Design review of the part built by this model. Coordinates are the model's own, in mm. Face numbers are marked on the shaded views. Round coordinates to 2 decimals unless told otherwise and drop trailing zeros. Order: outer loops, then holes, each group sorted by start corner. A loop starts at its lowest first (then second) coordinate and runs counter-clockwise, first axis right, second up. Notation, with made-up numbers: (32.5, 41.25) - (69.5, 41.25) arc R12 cw to (69.5, 61.25) - close; hole circle Ø3 at (11, 16.25). An arc over 180 degrees is marked (long way). Use CSV: the item, a comma, the result in double quotes.
from build123d import *

# Parameters (mm, degrees)
BOSS_EXTRUDE1_DEPTH = 0.6
FILLET3_R           = 0.03
FILLET4_R           = 0.17
SCALE2_SCALE        = 10
SKETCH4_R           = 0.5334
SKETCH4_R_2         = 2
CUT_EXTRUDE5_DEPTH  = 1
SKETCH4_3_R         = 0.5334
SKETCH4_3_R_2       = 2
CUT_EXTRUDE6_DEPTH  = 0.5


with BuildPart() as part:
    # Sketch1 → Boss-Extrude1 (new body)
    with BuildSketch(Plane.XY):
        with BuildLine():
            Line((-0.136993219, -2.45), (0.163006781, -2.450375949))
            Line((0.163006781, -2.450375949), (0.499999859, -0.000375949))
            ThreePointArc((0.499999859, -0.000375949), (0.000187974, 0.499999965), (-0.5, 0))
            Line((-0.5, 0), (-0.136993219, -2.45))
        make_face()
    extrude(amount=BOSS_EXTRUDE1_DEPTH)

    # Fillet3
    fillet3_edges = [part.edges().sort_by_distance(p)[0] for p in [
        (0.33150332, -1.225375949, 0.6),
        (0.000187974, 0.499999965, 0.6),
        (-0.318496609, -1.225, 0.6),
        (0.000187974, 0.499999965, 0),
        (0.33150332, -1.225375949, 0),
        (0.013006781, -2.450187974, 0),
        (-0.318496609, -1.225, 0),
        (0.013006781, -2.450187974, 0.6),
    ]]
    fillet(fillet3_edges, radius=FILLET3_R)

    # Fillet4
    # the kernel refuses this fillet: 0.17 mm, written as the material it takes off along each edge
    with BuildSketch(Plane(origin=(0.009701663, -2.280183699, 0), x_dir=(-0.001253160871338018, -0.9999992147936071, 0), z_dir=(0.9999992147936071, -0.001253160871338018, 0))) as fillet4_piece_1:
        with BuildLine():
            CenterArc((0.14, -0.03), 0.03, 0, 90)
            Line((0.17, -0.03), (0.17, 0))
            Line((0.17, 0), (0.14, 0))
        make_face()
    revolve(axis=Axis((0.009701663, -2.280183699, 0), (0, 0, -1)), revolution_arc=81.500227405, mode=Mode.SUBTRACT)
    with BuildSketch(Plane(origin=(0.014814914, -2.280190107, 0), x_dir=(0.9906723955714478, -0.1362651997126514, 0), z_dir=(0.1362651997126514, 0.9906723955714478, 0))) as fillet4_piece_2:
        with BuildLine():
            CenterArc((0.14, -0.03), 0.03, 0, 90)
            Line((0.17, -0.03), (0.17, 0))
            Line((0.17, 0), (0.14, 0))
        make_face()
    revolve(axis=Axis((0.014814914, -2.280190107, 0), (0, 0, -1)), revolution_arc=82.240014231, mode=Mode.SUBTRACT)
    with BuildSketch(Plane(origin=(0.014814914, -2.280190107, 0.6), x_dir=(-0.001253160871338018, -0.9999992147936071, 0), z_dir=(-0.9999992147936071, 0.001253160871338018, 0))) as fillet4_piece_3:
        with BuildLine():
            CenterArc((0.14, -0.03), 0.03, 0, 90)
            Line((0.17, -0.03), (0.17, 0))
            Line((0.17, 0), (0.14, 0))
        make_face()
    revolve(axis=Axis((0.014814914, -2.280190107, 0.6), (0, 0, 1)), revolution_arc=82.240014231, mode=Mode.SUBTRACT)
    with BuildSketch(Plane(origin=(0.009701663, -2.280183699, 0.6), x_dir=(-0.9892008974747571, -0.14656597297850232, 0), z_dir=(-0.14656597297850232, 0.9892008974747571, 0))) as fillet4_piece_4:
        with BuildLine():
            CenterArc((0.14, -0.03), 0.03, 0, 90)
            Line((0.17, -0.03), (0.17, 0))
            Line((0.17, 0), (0.14, 0))
        make_face()
    revolve(axis=Axis((0.009701663, -2.280183699, 0.6), (0, 0, 1)), revolution_arc=81.500227405, mode=Mode.SUBTRACT)
    with BuildSketch(Plane(origin=(0.163006781, -2.450375949, 0), x_dir=(-0.999999214793607, 0.001253160871339251, 0), z_dir=(0, 0, 1))) as fillet4_piece_5:
        with BuildLine():
            CenterArc((FILLET4_R * 0.872970713312, -FILLET4_R), FILLET4_R, 90, 82.240014231)
            Line((-FILLET4_R * 0.117871666593, -FILLET4_R * 0.864976379166), (0, 0))
            Line((0, 0), (FILLET4_R * 0.872970713312, 0))
        make_face()
    extrude(amount=0.6, mode=Mode.SUBTRACT)
    with BuildSketch(Plane(origin=(-0.136993219, -2.45, 0), x_dir=(-0.14656597297850246, 0.9892008974747571, 0), z_dir=(0, 0, 1))) as fillet4_piece_6:
        with BuildLine():
            CenterArc((FILLET4_R * 0.861658584387, -FILLET4_R), FILLET4_R, 90, 81.500227405)
            Line((-FILLET4_R * 0.127357865618, -FILLET4_R * 0.852194514247), (0, 0))
            Line((0, 0), (FILLET4_R * 0.861658584387, 0))
        make_face()
    extrude(amount=0.6, mode=Mode.SUBTRACT)


with BuildPart() as part_1:
    # Scale2: scaled about (0.00425557, -0.756697726, 0.299999998)
    add(part.part.scale(SCALE2_SCALE).moved(Location((-0.03830013, 6.810279534, -2.699999982))))

    # Sketch4 → Cut-Extrude5 (cut)
    with BuildSketch(Plane(origin=(0, 0, -2.70000001), x_dir=(-1, 0, 0), z_dir=(0, 0, -1))):
        with Locations((0.041676609, 0.695226981)):
            Circle(SKETCH4_R)
        with Locations((0.042616275, -1.00657276)):
            Circle(SKETCH4_R)
        with Locations((0.04355594, -2.7083725)):
            Circle(SKETCH4_R)
        with Locations((0.044495606, -4.410172241)):
            Circle(SKETCH4_R)
        with Locations((0.045435271, -6.111971981)):
            Circle(SKETCH4_R)
        with Locations((0.046374936, -7.813771722)):
            Circle(SKETCH4_R)
        with Locations((0.038300124, 6.810276049)):
            Circle(SKETCH4_R_2)
    extrude(amount=-CUT_EXTRUDE5_DEPTH, mode=Mode.SUBTRACT)

    # Sketch4<3> → Cut-Extrude6 (cut)
    with BuildSketch(Plane(origin=(0, 0, -2.70000001), x_dir=(-1, 0, 0), z_dir=(0, 0, -1))):
        with BuildLine():
            Line((1.792330148, -7.279407594), (2.852562233, 4.61584025))
            ThreePointArc((2.852562233, 4.61584025), (0.036329632, 10.378975505), (-2.77353691, 4.612733744))
            Line((-2.77353691, 4.612733744), (-1.700169319, -7.281336012))
            ThreePointArc((-1.700169319, -7.281336012), (0.047044623, -9.026621537), (1.792330148, -7.279407594))
        make_face()
        with Locations((0.041676609, 0.695226981)):
            Circle(SKETCH4_3_R, mode=Mode.SUBTRACT)
        with Locations((0.042616275, -1.00657276)):
            Circle(SKETCH4_3_R, mode=Mode.SUBTRACT)
        with Locations((0.04355594, -2.7083725)):
            Circle(SKETCH4_3_R, mode=Mode.SUBTRACT)
        with Locations((0.044495606, -4.410172241)):
            Circle(SKETCH4_3_R, mode=Mode.SUBTRACT)
        with Locations((0.045435271, -6.111971981)):
            Circle(SKETCH4_3_R, mode=Mode.SUBTRACT)
        with Locations((0.046374936, -7.813771722)):
            Circle(SKETCH4_3_R, mode=Mode.SUBTRACT)
        with Locations((0.038300124, 6.810276049)):
            Circle(SKETCH4_3_R_2, mode=Mode.SUBTRACT)
    extrude(amount=-CUT_EXTRUDE6_DEPTH, mode=Mode.SUBTRACT)


solid = part_1.part
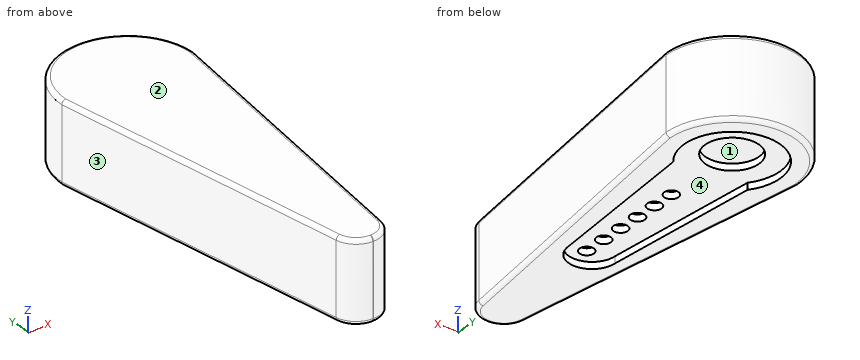
1) Insertion check: pin 1 Ø0.6 at (x, y) = (-0.04, 0.7) entering from -Z; pin 2 Ø1 at (x, z) = (-2.5, 1) entering from +Y; pin 3 Ø1.2 at (x, y) = (-0.5, -6.5) entering from -Z. Each pin has a flat end and moves straight along its axis. Give the tip position at first contact, or say it passes through.
Data:
pin 1,"stops at z = -1.7"
pin 2,"stops at y = 11.41"
pin 3,"stops at z = -2.2"
2) The part is to be moulded in two halves that separate along Y. For the marked faces 1, 2, 3 and 4, say which applies: +Y half, -Y half, draft (parallel to the pull), parting line (faces both ways), or undercut.
Data:
face 1,"undercut"
face 2,"draft"
face 3,"-Y half"
face 4,"undercut"
3) To check wall thickness, follow L1, parallel to X at y = 7.25, z = -2.25; L2, parallel to X at y = 7, z = 1.5; L3, parallel to Z at x = 1.75, y = 6.75. State the ranges of each line that lie inside material, in increasing order. Write a range as from..to.
Data:
L1,"x = -5.02..-3.58, 3.5..4.94"
L2,"x = -5.03..4.96"
L3,"z = -1.7..3.3"
4) We need section A-A (z = 0.5). Give the boundary of the cut face in (x, y).
Data:
outline,"(-5.04, 6.81) - (-1.62, -16.24) arc R1.7 ccw to (0.06, -17.69) - (0.11, -17.69) arc R1.7 ccw to (1.79, -16.22) - (4.96, 6.81) arc R5 ccw to start"
